The listing builds one solid part. Answer for the finished solid, in the listing's coordinates (mm). Face numbers are marked on the shaded views. A direction names the side the tool comes from. Round coordinates to 2 decimals unless told otherwise and drop trailing zeros. Order: outer loops, then holes, each group sorted by start corner. A loop starts at its lowest first (then second) coordinate and runs counter-clockwise, first axis right, second up. Notation, with made-up numbers: (-22, 75) -> (8, 75) arc R20 cw to (8, 114) -> close; hole circle Ø11 at (68, 64.5). An arc over 180 degrees is marked (long way). Return JSON: item names as keys, results as strings. Group by question number.
(1) The part is cut by section B-B (x = 55). Determine the outline of the cut face in (y, z), plus the area to 3 significant figures.
(2) The part is cut by section C-C (z = 5.5). Determine the outline of the cut face in (x, y), plus the area to 3 significant figures.
(3) Which of the six approach directions +Z, -Z, +X, -X, +Y, -Y give full straight-line access (tool end or side, diameter ignored) to the marked faces 1, 2 and 3?
(4) The part is cut by section D-D (y = -41.5). Determine the outline of the cut face in (x, z), plus the area to 3 significant figures.
(5) Each of these flat-tipped pins is pushed along its axis until it touches: pin 1 (8 mm diameter, centred on y = -7, z = 14, fed in from +X); pin 2 (2 mm diameter, centred on x = 15.5, y = -37.5, fed in from +Z); pin 3 (4 mm diameter, centred on x = 15, z = 8, fed in from +Y); pin 4 (7 mm diameter, centred on x = 55.5, y = 2, fed in from +Z). Where does it stop, or does it pass through?
(6) Consider line 1 (X direction, y = -1.95, z = 12.65); line 2 (Z direction, x = 27.5, y = 2.5); line 3 (Y direction, x = 73, z = 12.25). Determine where each line is inside the solid, lowest interval first. Write a range as [from, to].
(7) The part is cut by section A-A (z = 12.65). Determine the outline of the cut face in (x, y), plus the area to 3 significant figures.
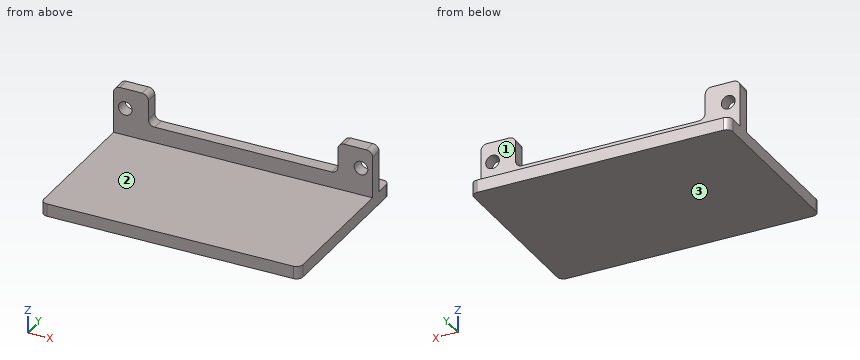
from build123d import *

# Parameters (mm, degrees)
SKETCH1_W           = 82
SKETCH1_H           = 49
BOSS_EXTRUDE1_DEPTH = 4
SKETCH2_W           = 82
SKETCH2_H           = 4
BOSS_EXTRUDE2_DEPTH = 15
SKETCH3_R           = 2.159
CUT_EXTRUDE1_DEPTH  = 50
SKETCH4_W           = 82
SKETCH4_H           = 4
BOSS_EXTRUDE3_DEPTH = 6.35
SKETCH5_W           = 60
SKETCH5_H           = 4
CUT_EXTRUDE2_DEPTH  = 10
FILLET1_R           = 2


with BuildPart() as part:
    # Sketch1 → Boss-Extrude1 (new body)
    with BuildSketch(Plane.XY):
        with Locations((41, -24.5)):
            Rectangle(SKETCH1_W, SKETCH1_H)
    extrude(amount=BOSS_EXTRUDE1_DEPTH)

    # Sketch2 → Boss-Extrude2 (add)
    with BuildSketch(Plane.XY.offset(4)):
        with Locations((41, -2)):
            Rectangle(SKETCH2_W, SKETCH2_H)
    extrude(amount=BOSS_EXTRUDE2_DEPTH)

    # Sketch3 → Cut-Extrude1 (cut, through all)
    with BuildSketch(Plane(origin=(0, 0, 0), x_dir=(1, 0, 0), z_dir=(0, 1, 0))):
        with Locations((3.704833995, -12.65)):
            Circle(SKETCH3_R)
        with Locations((78.295166005, -12.65)):
            Circle(SKETCH3_R)
    extrude(amount=-CUT_EXTRUDE1_DEPTH, mode=Mode.SUBTRACT)

    # Sketch4 → Boss-Extrude3 (add)
    with BuildSketch(Plane(origin=(0, 0, 0), x_dir=(1, 0, 0), z_dir=(0, 1, 0))):
        with Locations((41, -2)):
            Rectangle(SKETCH4_W, SKETCH4_H)
    extrude(amount=BOSS_EXTRUDE3_DEPTH)

    # Sketch5 → Cut-Extrude2 (cut)
    with BuildSketch(Plane.XY.offset(19)):
        with Locations((41, -2)):
            Rectangle(SKETCH5_W, SKETCH5_H)
    extrude(amount=-CUT_EXTRUDE2_DEPTH, mode=Mode.SUBTRACT)

    # Fillet1
    fillet1_edges = [part.edges().sort_by_distance(p)[0] for p in [
        (0, -2, 19),
        (82, -2, 19),
        (0, 6.35, 2),
        (82, 6.35, 2),
        (71, -2, 9),
        (11, -2, 9),
        (71, -2, 19),
        (11, -2, 19),
        (82, -49, 2),
        (0, -49, 2),
    ]]
    fillet(fillet1_edges, radius=FILLET1_R)


solid = part.part
Answer below:
{
 "1": {"outline": "(-49, 0) -> (6.35, 0) -> (6.35, 4) -> (0, 4) -> (0, 9) -> (-4, 9) -> (-4, 4) -> (-49, 4) -> close", "area": "241 mm²"},
 "2": {"outline": "(0, -4) -> (82, -4) -> (82, 0) -> (0, 0) -> close", "area": "328 mm²"},
 "3": {"face 1": "+Z, +X, -X, +Y", "face 2": "+Z, +X, -X, -Y", "face 3": "-Z, +X, -X, +Y, -Y"},
 "4": {"outline": "(0, 0) -> (82, 0) -> (82, 4) -> (0, 4) -> close", "area": "328 mm²"},
 "5": {"pin 1": "stops at x = 82", "pin 2": "stops at z = 4", "pin 3": "stops at y = 0", "pin 4": "stops at z = 9"},
 "6": {"line 1": "x = [0, 1.55], [5.86, 11], [71, 76.14], [80.45, 82]", "line 2": "z = [0, 4]", "line 3": "y = [-4, 0]"},
 "7": {"outline": "(0, -4) -> (1.55, -4) -> (1.55, 0) -> (0, 0) -> close; (5.86, -4) -> (11, -4) -> (11, 0) -> (5.86, 0) -> close; (71, -4) -> (76.14, -4) -> (76.14, 0) -> (71, 0) -> close; (80.45, -4) -> (82, -4) -> (82, 0) -> (80.45, 0) -> close", "area": "53.5 mm²"}
}
